Can you work these out from the model? Positions are in its coordinate system, mm. A direction names the side the tool comes from. Give positions to 0.01 mm unless a question says otherwise; leave off trailing zeros. Write each loop counter-clockwise with the first axis right and the second up, starting at its lowest first coordinate (ties: lowest second). Pieces come first, ordered by that corner, then holes. Notation, with made-up numbers: M 32,21.25 L 82,21.25 A12 ccw 82,31.25 Z; hole C 79,-14.5 d6. An arc over 180 degrees is marked long. Answer as CSV lines item,"result". Start each with the question number.
```python
from build123d import *

# Parameters (mm, degrees)
SKETCH1_W           = 94.107
SKETCH1_H           = 127
BOSS_EXTRUDE1_DEPTH = 6
SKETCH2_W           = 5.9944
SKETCH2_H           = 9.779
CUT_EXTRUDE1_DEPTH  = 159.180679759
SKETCH3_R           = 1.27
CUT_EXTRUDE2_DEPTH  = 159.180679759
SKETCH4_R           = 4.0005
SKETCH4_W           = 19.304
SKETCH4_H           = 12.7
CUT_EXTRUDE3_DEPTH  = 159.180679759
SKETCH5_R           = 1.4605
CUT_EXTRUDE4_DEPTH  = 159.180679759


with BuildPart() as part:
    # Sketch1 → Boss-Extrude1 (new body)
    with BuildSketch(Plane.XY):
        with Locations((47.0535, 63.5)):
            Rectangle(SKETCH1_W, SKETCH1_H)
    extrude(amount=BOSS_EXTRUDE1_DEPTH)

    # Sketch2 → Cut-Extrude1 (cut, through all)
    with BuildSketch(Plane.XY.offset(6)):
        with Locations((2.9972, 103.0605)):
            Rectangle(SKETCH2_W, SKETCH2_H)
        with Locations((91.1098, 103.0605)):
            Rectangle(SKETCH2_W, SKETCH2_H)
        with Locations((2.9972, 33.2105)):
            Rectangle(SKETCH2_W, SKETCH2_H)
        with Locations((91.1098, 33.2105)):
            Rectangle(SKETCH2_W, SKETCH2_H)
    extrude(amount=-CUT_EXTRUDE1_DEPTH, mode=Mode.SUBTRACT)

    # Sketch3 → Cut-Extrude2 (cut, through all)
    with BuildSketch(Plane(origin=(0, 0, 0), x_dir=(-1, 0, 0), z_dir=(0, 0, -1))):
        with Locations((-67.31, 24.384)):
            Circle(SKETCH3_R)
        with Locations((-67.31, 116.84)):
            Circle(SKETCH3_R)
        with Locations((-13.97, 116.84)):
            Circle(SKETCH3_R)
        with Locations((-13.97, 24.384)):
            Circle(SKETCH3_R)
    extrude(amount=-CUT_EXTRUDE2_DEPTH, mode=Mode.SUBTRACT)

    # Sketch4 → Cut-Extrude3 (cut, through all)
    with BuildSketch(Plane.XY.offset(6)):
        with Locations((37.0586, 9.525)):
            Circle(SKETCH4_R)
        with Locations((65.7606, 12.7)):
            Rectangle(SKETCH4_W, SKETCH4_H)
    extrude(amount=-CUT_EXTRUDE3_DEPTH, mode=Mode.SUBTRACT)

    # Sketch5 → Cut-Extrude4 (cut, through all)
    with BuildSketch(Plane.XY.offset(6)):
        with Locations((2.9972, 76.2)):
            Circle(SKETCH5_R)
        with Locations((91.1098, 76.2)):
            Circle(SKETCH5_R)
    extrude(amount=-CUT_EXTRUDE4_DEPTH, mode=Mode.SUBTRACT)


solid = part.part
```
1) I want a section at C-C, the plane x = 37.5. Please give me the cut outline in (y, z).
2) I want a section at D-D, the plane z = 4.75. State how many separate pieces and enclosed holes the cut face has, then the cut area to 3 significant figures.
3) I want a section at A-A, the plane y = 116.84. Please give me the cut outline in (x, z).
4) I want a section at B-B, the plane x = 13.97. Please give me the cut outline in (y, z), then the cut area to 3 significant figures.
5) Thinking about a two-plate mould opening in X: for faces 1 (the flat face through (0, 117, 3)), 2 (the flat face through (88.113, 33, 3)), 3 (the flat face through (66, 19.05, 3)), which applies, released by +X, released by -X, zero draft, split by the parting line, or undercut?
6) On a 3-axis mill with a long thin cutter (end or side, diameter ignored), from which of +Z, -Z, +X, -X, +Y, -Y can I reach the whole of each face in a straight line? I mean faces 4 (the flat face through (5.994, 103, 3)), 5 (the cylindrical face through (14.245, 23.144, 2.958)), 6 (the flat face through (91, 38.1, 3)). Say none if no direction works.
7) I need wall thicknesses on L1, parallel to X at y = 76.2, z = 1.7; L2, parallel to Y at x = 67.31, z = 3.85; L3, parallel to Y at x = 57, z = 5.6. Which ranges of each line are inside material? Lowest first, please. Write a range as from..to.
8) I'm going to push flat-ended pins straight in: P1, Ø8, axis at x = 12, y = 48, coming from the -Z side; P2, Ø3, axis at y = 34.5, z = 3.5, coming from the -X side; P3, Ø1.8, axis at y = 34, z = 3, coming from the +X side; P4, Ø8, axis at x = 64.5, y = 14, coming from the -Z side. Where does each tip first touch, or does it pass through?
Values found:
1,outline,"M 0,0 L 5.55,0 L 5.55,6 L 0,6 Z; M 13.5,0 L 127,0 L 127,6 L 13.5,6 Z"
2,separate pieces,"1"
2,enclosed holes,"8"
2,area,"11,400 mm²"
3,outline,"M 0,0 L 12.7,0 L 12.7,6 L 0,6 Z; M 15.24,0 L 66.04,0 L 66.04,6 L 15.24,6 Z; M 68.58,0 L 94.11,0 L 94.11,6 L 68.58,6 Z"
4,outline,"M 0,0 L 23.11,0 L 23.11,6 L 0,6 Z; M 25.65,0 L 115.57,0 L 115.57,6 L 25.65,6 Z; M 118.11,0 L 127,0 L 127,6 L 118.11,6 Z"
4,area,"732 mm²"
5,face 1,"released by -X"
5,face 2,"released by +X"
5,face 3,"undercut"
6,face 4,"+Z, -Z, -X"
6,face 5,"+Z, -Z"
6,face 6,"+Z, -Z, +X"
7,L1,"x = 0..1.54, 4.46..89.65, 92.57..94.11"
7,L2,"y = 0..6.35, 19.05..23.11, 25.65..115.57, 118.11..127"
7,L3,"y = 0..6.35, 19.05..127"
8,P1,"stops at z = 0"
8,P2,"stops at x = 5.99"
8,P3,"stops at x = 88.11"
8,P4,"passes through"
